The model under review builds one solid part; all positions refer to its coordinate system, in mm. A direction names the side the tool comes from. Coordinates: 2 decimals unless noted, no trailing zeros. Order: outer loops, then holes, each group sorted by start corner. A loop starts at its lowest first (then second) coordinate and runs counter-clockwise, first axis right, second up.
```python
from build123d import *

# Parameters (mm, degrees)
SKETCH_1_W          = 3
SKETCH_1_H          = 10
SKETCH_1_W_2        = 74
SKETCH_1_H_2        = 18
EXTRUDE_1_DEPTH     = 3
SKETCH_2_W          = 3
SKETCH_2_H          = 10
CUT_EXTRUDE_1_DEPTH = 3


with BuildPart() as part:
    # 草圖1 → 填料-伸長1 (new body)
    with BuildSketch(Plane.XY):
        with Locations((-38.5, 0)):
            Rectangle(SKETCH_1_W, SKETCH_1_H)
        Rectangle(SKETCH_1_W_2, SKETCH_1_H_2)
        with Locations((38.5, 0)):
            Rectangle(SKETCH_1_W, SKETCH_1_H)
    extrude(amount=EXTRUDE_1_DEPTH)

    # 草圖2 → 除料-伸長1 (cut)
    with BuildSketch(Plane.XY.offset(3)):
        Rectangle(SKETCH_2_W, SKETCH_2_H)
    extrude(amount=-CUT_EXTRUDE_1_DEPTH, mode=Mode.SUBTRACT)


solid = part.part
```
(1) Draft analysis for pull direction X (two halves, no side actions). For faces 6 (the face through (0, 5, 2)), 7 (the face through (38, 5, 1)), 8 (the face through (37, 7, 1)), state which applies: released by +X, released by -X, zero draft, split by the parting line, or undercut.
A:
face 6: undercut
face 7: zero draft
face 8: released by +X
(2) Machinability: for faces 1 (the face through (-1.5, 0, 2)), 2 (the face through (-39, 5, 1)), 3 (the face through (38, -5, 1)), 4 (the face through (-39, -5, 1)), 5 (the face through (-1, -6, 0)), which of the approach directions +Z, -Z, +X, -X, +Y, -Y give a long, thin tool a straight path to every point of the face, cutting with its end or side? Answer none if there is none.
A:
face 1: +Z, -Z
face 2: +Z, -Z, -X, +Y
face 3: +Z, -Z, +X, -Y
face 4: +Z, -Z, -X, -Y
face 5: -Z, +X, -X, +Y, -Y
(3) We need section B-B, the plane y = 2. Write out the cut boundary in (x, z), and give its area (3 significant figures).
A:
outline: (-40, 0) - (-1.5, 0) - (-1.5, 3) - (-40, 3) - close; (1.5, 0) - (40, 0) - (40, 3) - (1.5, 3) - close
area: 231 mm2
(4) We need section C-C, the plane y = 6.75. Write out the cut boundary in (x, z), and give its area (3 significant figures).
A:
outline: (-37, 0) - (37, 0) - (37, 3) - (-37, 3) - close
area: 222 mm2
(5) We need section A-A, the plane z = 2.1. Write out the cut boundary in (x, y), and give its area (3 significant figures).
A:
outline: (-40, -5) - (-37, -5) - (-37, -9) - (37, -9) - (37, -5) - (40, -5) - (40, 5) - (37, 5) - (37, 9) - (-37, 9) - (-37, 5) - (-40, 5) - close; hole (-1.5, -5) - (1.5, -5) - (1.5, 5) - (-1.5, 5) - close
area: 1,360 mm2
(6) For pin 1 Ø1.5 at (y, z) = (-6.5, 1) entering from +X; pin 2 Ø1.5 at (x, z) = (-38.5, 1.5) entering from +Y; pin 3 Ø1.5 at (y, z) = (6, 1.5) entering from -X, all flat-tipped, find the tip position at first contact; note any pin that passes through.
A:
pin 1: stops at x = 37
pin 2: stops at y = 5
pin 3: stops at x = -37
(7) Wall thickness on probe 1 along X at (y, z) = (-1, 1); probe 2 along X at (y, z) = (6.75, 2.35): over which ranges is each line inside the solid? List them lowest first.
A:
probe 1: x = -40 to -1.5, 1.5 to 40
probe 2: x = -37 to 37
